```python
from build123d import *

# Parameters (mm, degrees)
F0_R      = 35
F1_DEPTH  = 5
F1_FACE_R = 35
F2_DEPTH  = 40
F2_TAPER  = -10
F3_DEPTH  = 10
F4_T      = -3


with BuildPart() as f1:
    # F0 (on Top) → F1 (new body)
    with BuildSketch(Plane.XY):
        Circle(F0_R)
    extrude(amount=-F1_DEPTH)

    # F1_face (on face) → F2 (join)
    with BuildSketch(Plane.XY):
        Circle(F1_FACE_R)
    extrude(amount=F2_DEPTH, taper=F2_TAPER)

    # F3 (add): a face of the model
    f3_faces = [f1.faces().sort_by_distance(p)[0] for p in [
        (0, 0, 40),
    ]]
    extrude(f3_faces, amount=F3_DEPTH)

    # F4
    f4_openings = [f1.faces().sort_by_distance(p)[0] for p in [
        (0, 0, 50),
    ]]
    offset(amount=F4_T, openings=f4_openings, kind=Kind.INTERSECTION)


solid = f1.part
```
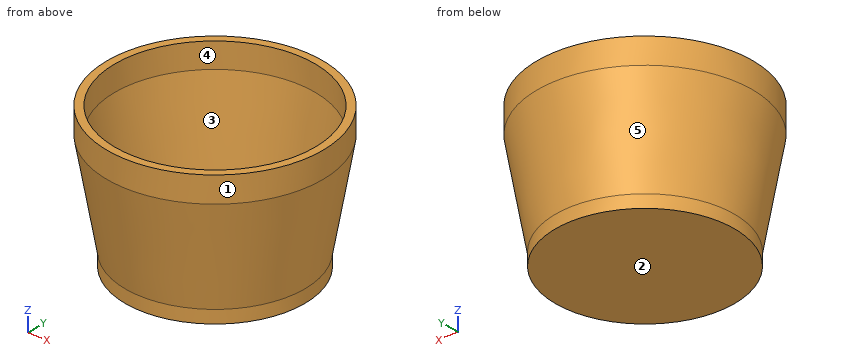
Geometry check sheet. Reference: the model listing, model coordinates, mm. Face numbers are marked on the shaded views. A direction names the side the tool comes from. Round coordinates to 2 decimals unless told otherwise and drop trailing zeros. Loops run counter-clockwise (first coordinate to the right, second up) from the corner with the lowest first, then second, coordinate; pieces in that order, holes last. Notation, with made-up numbers: (19.5, 28) - (51.5, 28) arc R23 ccw to (51.5, 57) - close; hole circle Ø4 at (-24.75, -9). An arc over 180 degrees is marked (long way). Write each question's results on one line, items separated by ' | '. Start each with the question number.
Q1. Gauge pin test, flat ends, axial feed: P1, Ø1, axis at y = 5.5, z = 38, coming from the +X side; P2, Ø1, axis at x = -12.5, z = 13.5, coming from the -Y side; P3, Ø8, axis at y = 1.5, z = 21.5, coming from the -X side. Record the tip position at first contact, or that the pin passes through.
Q2. Cross-section at C-C on z = 15. Enter the section's corners in (x, y).
Q3. Cross-section at B-B on z = 44. Enter the section's corners in (x, y).
Q4. Cross-section at A-A on x = 0. Enter the section's corners in (y, z).
Q5. Thickness scan on line 1 (Y direction, x = 0, z = 45.25); line 2 (Z direction, x = 14, y = 6); line 3 (Y direction, x = 0, z = -0.8). Record the ranges inside material, lowest first. Write a range as [from, to].
Q6. Access from +Z, -Z, +X, -X, +Y, -Y to the whole of each face (thin tool, end or side, straight path). Record for the marked faces 4 and 5.
Q7. Release check for a two-part mould opening along X. For the marked faces 1, 2 and 3 record: +X half, -X half, draft (parallel to the pull), parting line (faces both ways), or undercut.
Answers below:
1) P1: stops at x = 41.45 | P2: stops at y = -35.43 | P3: stops at x = -39.48
2) outline: circle Ø75.29 at (0, 0); hole circle Ø69.2 at (0, 0)
3) outline: circle Ø84.11 at (0, 0); hole circle Ø78.11 at (0, 0)
4) outline: (-42.05, 40) - (-35, 0) - (-35, -5) - (35, -5) - (35, 0) - (42.05, 40) - (42.05, 50) - (39.05, 50) - (39.05, 40.26) - (32, 0.26) - (32, -2) - (-32, -2) - (-32, 0.26) - (-39.05, 40.26) - (-39.05, 50) - (-42.05, 50) - close
5) line 1: y = [-42.05, -39.05], [39.05, 42.05] | line 2: z = [-5, -2] | line 3: y = [-35, -32], [32, 35]
6) face 4: +Z | face 5: -Z
7) face 1: parting line | face 2: draft | face 3: undercut
